CAD build for the part. Positions are in the model's coordinates, mm. Round coordinates to 2 decimals unless told otherwise and drop trailing zeros. Write each loop counter-clockwise with the first axis right and the second up, starting at its lowest first coordinate (ties: lowest second). Pieces come first, ordered by that corner, then holes. Notation, with made-up numbers: M 46.5,54 L 60.5,54 A26 cw 60.5,75 Z; hole C 7.5,26 d1. An arc over 180 degrees is marked long. Write each question's results on one line, items separated by ' | '. Start each with the question number.
Autodesk Inventor part; units mm, degrees
ref_plane "Work Plane1" through (6.4515, 0, 0) normal (0, 0.866, -0.5) x (-1, 0, 0)
ref_plane "YZ Plane" through (0, 0, 0) normal (1, 0, 0) x (0, 1, 0)
ref_plane "XZ Plane" through (0, 0, 0) normal (0, 1, 0) x (-1, 0, 0)
sketch "Skizze1" plane through (0, 0, 0) normal (1, 0, 0) x (0, 1, 0)
  line L0 (-4.6188, -8) -> (-9.2376, 0)
  line L1 (-9.2376, 0) -> (-4.6188, 8)
  line L2 (-4.6188, 8) -> (4.6188, 8)
  line L3 (4.6188, 8) -> (9.2376, 0)
  line L4 (9.2376, 0) -> (4.6188, -8)
  line L5 (4.6188, -8) -> (-4.6188, -8)
  point P0 (0, 0)
  point P1 (0, 0)
  dimension "d0" = 18.4752
extrude "Körper" add sketch "Skizze1" along normal blind 8
sketch "Skizze2" plane through (0, 0, 0) normal (0, 0, 1) x (1, 0, 0)
  line L0 (8, 0) -> (18, 0)
  arc A0 (18, 0) -> (10.5, 7.5) centre (10.5, 0) ccw
  line L1 (10.5, 7.5) -> (8, 7.5)
  line L2 (8, -4.6188) -> (8, 4.6188)
  line L3 (8, 0) -> (8, 7.5)
  line L4 (5.6893, 0) -> (21.864, 0)
  dimension "d8" = 7.5
  dimension "d9" = 10
revolve "Kopf" add sketch "Skizze2" angle 360 about axis through (8, 0, 0) along (1, 0, 0)
sketch "Skizze3" plane through (0, 0, 0) normal (-1, 0, 0) x (0, 0, 1)
  line L0 (0, -12.9326) -> (0, 12.9326)
  line L1 (-11.2, 0) -> (11.2, 0)
  point P0 (0, 0)
hole "Gewinde" at (0, 0, 0) direction (1, 0, 0) diameter 8.647 depth 12.903 tip angle 120
sketch "Skizze4" plane through (0, 0, 0) normal (0, 0, 1) x (1, 0, 0)
  line L0 (0, 4.6188) -> (0, 9.2376)
  line L1 (0, 9.2376) -> (8, 9.2376)
  line L2 (8, 4.6188) -> (8, 9.2376)
  line L3 (-1.6, 0) -> (9.6, 0)
  line L4 (1.1187, 9.2376) -> (0, 7.3)
  line L5 (7.2855, 9.2376) -> (8, 8)
  dimension "d3" = 14.6
  dimension "d4" = 30
  dimension "d5" = 16
  dimension "d6" = 30
revolve "Fase1" cut sketch "Skizze4" angle 360 about axis through (-10, 0, 0) along (1, 0, 0)
chamfer "Fase2" distance 0.6766 angle 30 1 edges at (0, 0, -4.3235) measured on face at (0, 6.2266, -0.756)
ref_plane "Work Plane1" through (6.4515, 0, 0) normal (0, 0.866, -0.5) x (-1, 0, 0)
equation "\"d0\" = 1.1547 * SW"
equation "\"d1\" = SIH"
equation "\"d8\" = KR"
equation "\"d9\" = KOH1 - SIH"
equation "\"d11\" = GEL"
equation "\"d12\" = 1.02 * GEL"
equation "\"d3\" = SW0"
equation "\"d4\" = ANG1"
equation "\"d5\" = SW01"
equation "\"d6\" = ANG2"
equation "\"d14\" = -0.5 * GD1 + 0.5 * NND"
equation "\"d36\" = -0.5 * GD1 + 0.5 * NND"
equation "\"ANG1\" = 30deg"
equation "\"ANG2\" = 30deg"
equation "\"SIH\" = 8"
equation "\"KOH1\" = 18"
equation "\"GEL\" = 12.65"
equation "\"SW\" = 16"
equation "\"KR\" = 7.5"
equation "\"SW0\" = 14.6"
equation "\"SW01\" = SW"
equation "\"GUL\" = 0.541266 * PTC"
equation "\"TOA\" = 30deg"
equation "\"PTC\" = 1.25"
equation "\"E0\" = 1.155 * SW"
equation "\"GAL\" = 0.541266 * PTC"
properties part number "DIN 1587 - M10 x 1,25 - SW16" material "Stahl, weich"
1) Saw through at A-A, the plane x = 4.25. Write the cut outline in (y, z).
2) Wall check: line 1 along Z through (x, y) = (5, 0); line 2 along Z through (x, y) = (10.5, 0); line 3 along X through (y, z) = (8, -0.25). Give the ranges that are in metal, low to high. Write a range as from..to.
3) Saw through at B-B, the plane x = 8.5. Write the cut outline in (y, z), plus the area to 3 significant figures.
4) Pull direction Y, two halves, no side cores. Call faces 1 (the face through (9.232, -7.493, -0.33)), 2 (the face through (14.97, -0.73, -0.16)), 3 (the face through (8, 5, -6)), 4 (the face through (6.73, 2.63, -3.43)): pulls with the +Y half, pulls with the -Y half, needs draft (parallel to the pull), parting line crosses it, or undercut.
5) Saw through at C-C, the plane x = 14. Write the cut outline in (y, z), plus the area to 3 significant figures.
6) Drop flat-ended pins along their axis: pin 1 Ø3 at (x, y) = (16, -0.5) entering from +Z; pin 2 Ø1 at (x, z) = (10.5, -5) entering from +Y; pin 3 Ø1.5 at (x, y) = (7.5, 6.5) entering from +Z. Give the stop position or say it passes through.
Filled sheet:
1) outline: M -9.24,0 L -4.62,-8 L 4.62,-8 L 9.24,0 L 4.62,8 L -4.62,8 Z; hole C 0,0 d8.65
2) line 1: z = -8..-4.32, 4.32..8 | line 2: z = -7.5..-4.32, 4.32..7.5 | line 3: x = 0.41..8
3) outline: C 0,0 d15; hole C 0,0 d8.65 | area: 118 mm^2
4) face 1: parting line crosses it | face 2: undercut | face 3: needs draft | face 4: undercut
5) outline: C 0,0 d13.27; hole C 0,0 d4.85 | area: 120 mm^2
6) pin 1: stops at z = 6.33 | pin 2: stops at y = 6 | pin 3: stops at z = 6.04
